Here's how the part is built. I have some questions about the finished solid (model axes, mm). A direction names the side the tool comes from. Round coordinates to 2 decimals unless told otherwise and drop trailing zeros. Write each loop counter-clockwise with the first axis right and the second up, starting at its lowest first coordinate (ties: lowest second). Pieces come first, ordered by that corner, then holes. Notation, with made-up numbers: (-32, 37) -> (2, 37) arc R16 ccw to (2, 52) -> close; hole circle Ø8 at (10, 87). An arc over 180 degrees is marked (long way). Put each result on its own line as item: value. Start each with the question number.
1) I want a section at B-B, the plane y = 35. List the corners of the cut face in (x, z) for me, then the cut area to 3 significant figures.
2) I want a section at D-D, the plane x = -13. List the corners of the cut face in (y, z) for me.
3) I want a section at C-C, the plane x = 70. List the corners of the cut face in (y, z) for me, then the cut area to 3 significant figures.
4) I want a section at A-A, the plane z = 5.5. List the corners of the cut face in (x, y) for me.
5) We'd pull the mould along Y, two halves only. Please class faces 1 (the flat face through (-75, 0, -5)), 2 (the cylindrical face through (1.12, 48.57, -6)), 3 (the cylindrical face through (-83.57, 0.63, -6)): released by +Y, released by -Y, zero draft, split by the parting line, or undercut.
6) Which directions (+Z, -Z, +X, -X, +Y, -Y) give clear straight access to the entire face, cutting with the end or side of a thin tool? Please do faces 4 (the flat face through (75, 0, -5)), 5 (the cylindrical face through (-72.21, -32.97, -0.11)).
7) If I drill on line 1 along Y through (x, z) = (70, 1); line 2 along Y through (x, z) = (70, -3.75); line 3 along X through (y, z) = (36, 0.5), over which ranges is the centre line in solid material (lowest first)? Write a range as [from, to].
8) Will these pins go through, and if not, where does the flat tip stop? P1, Ø1.5, axis at y = -8, z = -4, coming from the -X side; P2, Ø5, axis at x = -70, y = -35, coming from the +Z side; P3, Ø1.5, axis at x = -13, z = -4, coming from the -Y side; P4, Ø4, axis at x = 4, y = -30.5, coming from the -Z side.
from build123d import *

# Parameters (mm, degrees)
F0_W     = 170
F0_H     = 100
F0_R     = 3
F1_DEPTH = 7.5
F2_T     = -10
F3_R     = 5
F4_R     = 3
F5_DEPTH = 5


with BuildPart() as f1:
    # F0 (on Top) → F1 (new body, symmetric)
    with BuildSketch(Plane.XY):
        Rectangle(F0_W, F0_H)
        with Locations((-70, -35)):
            Circle(F0_R, mode=Mode.SUBTRACT)
        with Locations((70, -35)):
            Circle(F0_R, mode=Mode.SUBTRACT)
        with Locations((-70, 35)):
            Circle(F0_R, mode=Mode.SUBTRACT)
        with Locations((70, 35)):
            Circle(F0_R, mode=Mode.SUBTRACT)
    extrude(amount=F1_DEPTH, both=True)

    # F2
    f2_openings = [f1.faces().sort_by_distance(p)[0] for p in [
        (0, 0, -7.5),
    ]]
    offset(amount=F2_T, openings=f2_openings, kind=Kind.INTERSECTION)

    # F3
    f3_edges = [f1.edges().sort_by_distance(p)[0] for p in [
        (-85, 0, -7.5),
        (-85, 0, 7.5),
        (0, -50, 7.5),
        (0, -50, -7.5),
        (85, 0, -7.5),
        (85, 0, 7.5),
        (85, 50, 0),
        (0, 50, 7.5),
        (0, 50, -7.5),
        (-85, 50, 0),
        (-85, -50, 0),
        (85, -50, 0),
    ]]
    fillet(f3_edges, radius=F3_R)

    # F4 (on face) → F5 (join)
    with BuildSketch(Plane(origin=(0, 0, -2.5), x_dir=(1, 0, 0), z_dir=(0, 0, -1))):
        with BuildLine():
            Line((65, -40), (75, -40))
            Line((75, -40), (75, -30))
            ThreePointArc((75, -30), (65, -30), (65, -40))
        make_face()
        with Locations((70, -35)):
            Circle(F4_R, mode=Mode.SUBTRACT)
        with BuildLine():
            Line((-75, -30), (-75, -40))
            Line((-75, -40), (-65, -40))
            ThreePointArc((-65, -40), (-65, -30), (-75, -30))
        make_face()
        with Locations((-70, -35)):
            Circle(F4_R, mode=Mode.SUBTRACT)
        with BuildLine():
            Line((-65, 40), (-75, 40))
            Line((-75, 40), (-75, 30))
            ThreePointArc((-75, 30), (-65, 30), (-65, 40))
        make_face()
        with Locations((-70, 35)):
            Circle(F4_R, mode=Mode.SUBTRACT)
        with BuildLine():
            Line((75, 30), (75, 40))
            Line((75, 40), (65, 40))
            ThreePointArc((65, 40), (65, 30), (75, 30))
        make_face()
        with Locations((70, 35)):
            Circle(F4_R, mode=Mode.SUBTRACT)
    extrude(amount=F5_DEPTH)


solid = f1.part
Findings:
1. outline: (-85, -2.5) arc R5 ccw to (-80, -7.5) -> (-73, -7.5) -> (-73, 7.5) -> (-80, 7.5) arc R5 ccw to (-85, 2.5) -> close; (-67, -7.5) -> (-57, -7.5) -> (-57, -2.5) -> (57, -2.5) -> (57, -7.5) -> (67, -7.5) -> (67, 7.5) -> (-67, 7.5) -> close; (73, -7.5) -> (80, -7.5) arc R5 ccw to (85, -2.5) -> (85, 2.5) arc R5 ccw to (80, 7.5) -> (73, 7.5) -> close
1. area: 1,780 mm2
2. outline: (-50, -2.5) arc R5 ccw to (-45, -7.5) -> (-40, -7.5) -> (-40, -2.5) -> (40, -2.5) -> (40, -7.5) -> (45, -7.5) arc R5 ccw to (50, -2.5) -> (50, 2.5) arc R5 ccw to (45, 7.5) -> (-45, 7.5) arc R5 ccw to (-50, 2.5) -> close
3. outline: (-50, -2.5) arc R5 ccw to (-45, -7.5) -> (-38, -7.5) -> (-38, 7.5) -> (-45, 7.5) arc R5 ccw to (-50, 2.5) -> close; (-32, -7.5) -> (-22, -7.5) -> (-22, -2.5) -> (22, -2.5) -> (22, -7.5) -> (32, -7.5) -> (32, 7.5) -> (-32, 7.5) -> close; (38, -7.5) -> (45, -7.5) arc R5 ccw to (50, -2.5) -> (50, 2.5) arc R5 ccw to (45, 7.5) -> (38, 7.5) -> close
3. area: 1,080 mm2
4. outline: (-84, -45) arc R4 ccw to (-80, -49) -> (80, -49) arc R4 ccw to (84, -45) -> (84, 45) arc R4 ccw to (80, 49) -> (-80, 49) arc R4 ccw to (-84, 45) -> close; hole circle Ø6 at (-70, -35); hole circle Ø6 at (-70, 35); hole circle Ø6 at (70, -35); hole circle Ø6 at (70, 35)
5. face 1: undercut
5. face 2: released by +Y
5. face 3: zero draft
6. face 4: -Z
6. face 5: +Z, -Z
7. line 1: y = [-50, -38], [-32, 32], [38, 50]
7. line 2: y = [-49.84, -38], [-32, -22], [22, 32], [38, 49.84]
7. line 3: x = [-85, -72.83], [-67.17, 67.17], [72.83, 85]
8. P1: stops at x = -84.94
8. P2: passes through
8. P3: stops at y = -49.94
8. P4: stops at z = -2.5
